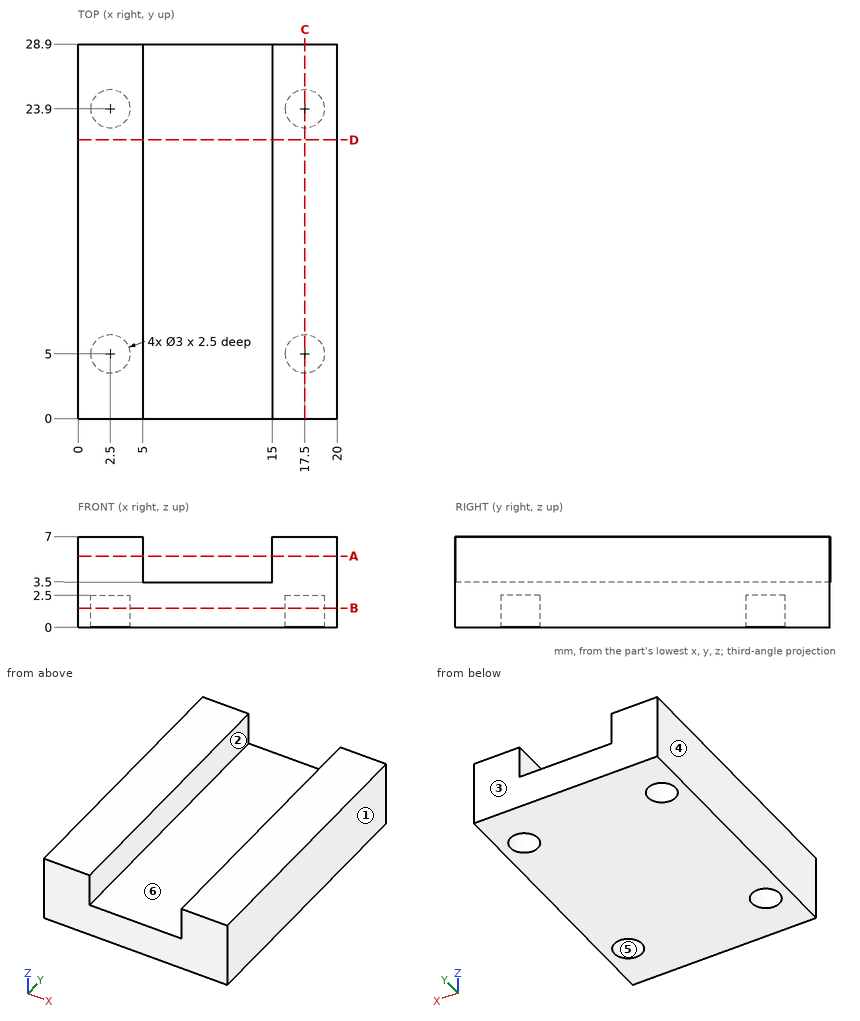
Source: three-view drawing plus pictorial views. Frame: mm from the lowest corner of the part. A direction names the side the tool comes from. Coordinates: 2 decimals unless noted, no trailing zeros. Loops run counter-clockwise (first coordinate to the right, second up) from the corner with the lowest first, then second, coordinate; pieces in that order, holes last. Notation, with made-up numbers: (5.25, -3.75) -> (21.25, -3.75) arc R23 ccw to (21.25, 26.25) -> close; hole circle Ø11 at (59, -21). An arc over 180 degrees is marked (long way). One line per item, written item: value.
(1) Ray query, line 1 along Y through (x, z) = (17.5, 1.45); line 2 along X through (y, z) = (26.75, 4.5); line 3 along Y through (x, z) = (3.5, 0.75). Return the intervals inside material, ascending.
Answer below:
line 1: y = 0 to 3.5, 6.5 to 22.4, 25.4 to 28.9
line 2: x = 0 to 5, 15 to 20
line 3: y = 0 to 3.88, 6.12 to 22.78, 25.02 to 28.9
(2) Pin query (flat end, axial travel): pin 1 Ø1.8 at (x, y) = (17.5, 5) entering from -Z; pin 2 Ø3 at (x, y) = (7.5, 18) entering from +Z. Return the tip coordinate at first contact, or that it passes through.
Answer below:
pin 1: stops at z = 2.5
pin 2: stops at z = 3.5
(3) Cut plane D-D (y = 21.5). Output: boundary loops of the cut face in (x, z), then the cut area to 3 significant figures.
Answer below:
outline: (0, 0) -> (20, 0) -> (20, 7) -> (15, 7) -> (15, 3.5) -> (5, 3.5) -> (5, 7) -> (0, 7) -> close
area: 105 mm2
(4) Cut plane B-B (z = 1.5). Output: boundary loops of the cut face in (x, y), then the cut area to 3 significant figures.
Answer below:
outline: (0, 0) -> (20, 0) -> (20, 28.9) -> (0, 28.9) -> close; hole circle Ø3 at (2.5, 5); hole circle Ø3 at (2.5, 23.9); hole circle Ø3 at (17.5, 5); hole circle Ø3 at (17.5, 23.9)
area: 550 mm2
(5) Draft query along X for the marked faces 1, 2 and 3. Return one class per face: pulls with the +X half, pulls with the -X half, needs draft (parallel to the pull), parting line crosses it, or undercut.
Answer below:
face 1: pulls with the +X half
face 2: undercut
face 3: needs draft
(6) Cut plane C-C (x = 17.5). Output: boundary loops of the cut face in (y, z), then the cut area to 3 significant figures.
Answer below:
outline: (0, 0) -> (3.5, 0) -> (3.5, 2.5) -> (6.5, 2.5) -> (6.5, 0) -> (22.4, 0) -> (22.4, 2.5) -> (25.4, 2.5) -> (25.4, 0) -> (28.9, 0) -> (28.9, 7) -> (0, 7) -> close
area: 187 mm2
(7) Cut plane A-A (z = 5.5). Output: boundary loops of the cut face in (x, y), then the cut area to 3 significant figures.
Answer below:
outline: (0, 0) -> (5, 0) -> (5, 28.9) -> (0, 28.9) -> close; (15, 0) -> (20, 0) -> (20, 28.9) -> (15, 28.9) -> close
area: 289 mm2
(8) Set-up query: the marked faces 4, 5 and 6. Return all of +Z, -Z, +X, -X, +Y, -Y with unobstructed straight access to the full face (end or side cutting, diameter ignored); none if empty.
Answer below:
face 4: +Z, -Z, -X, +Y, -Y
face 5: -Z
face 6: +Z, +Y, -Y
